Geometry check sheet. Reference: the model listing, model coordinates, mm. Face numbers are marked on the shaded views. A direction names the side the tool comes from. Give positions to 0.01 mm unless a question says otherwise; leave off trailing zeros. Write each loop counter-clockwise with the first axis right and the second up, starting at its lowest first coordinate (ties: lowest second). Pieces come first, ordered by that corner, then holes.
(1) Tool access check on the marked faces 1 and 2. Record the directions out of +Z, -Z, +X, -X, +Y, -Y that give a thin tool (end or side, any length) a straight path to the whole face; none if there is none.
(2) Thickness scan on line 1 along Y through (x, z) = (-10, -2); line 2 along X through (y, z) = (15, -73); line 3 along Z through (x, y) = (-15, 9.5). Record the ranges inside material, lowest first.
(3) Depth check by flat-ended pin: P1, Ø4, axis at x = -10, y = 10, coming from the -Z side; P2, Ø3, axis at y = 9.5, z = -33, coming from the +X side; P3, Ø12, axis at y = 9.5, z = -52.5, coming from the -X side; P4, Ø7, axis at x = -8, y = 11, coming from the -Z side. Enter the tip coordinate at first touch or a pass-through.
(4) Cross-section at B-B (x = -10). Record the boundary of the cut face in (y, z), and give its area (3 significant figures).
(5) Cross-section at D-D (x = 4). Record the boundary of the cut face in (y, z).
(6) Cross-section at C-C (z = -6). Record the boundary of the cut face in (x, y).
(7) Cross-section at A-A (y = 10). Record the boundary of the cut face in (x, z).
```python
from build123d import *

# Parameters (mm, degrees)
BOSS_EXTRUDE1_DEPTH = 20
SKETCH2_R           = 2.65
CUT_EXTRUDE1_DEPTH  = 20
SKETCH3_R           = 2.65
CUT_EXTRUDE2_DEPTH  = 20
SKETCH7_R           = 6
CUT_EXTRUDE4_DEPTH  = 5
SKETCH8_R           = 6
CUT_EXTRUDE5_DEPTH  = 5
CHAMFER3_SIZE       = 4
FILLET2_R           = 4
CHAMFER4_SIZE       = 2
CHAMFER5_SIZE       = 1


with BuildPart() as part:
    # Sketch1 → Boss-Extrude1 (new body)
    with BuildSketch(Plane(origin=(0, 0, 0), x_dir=(1, 0, 0), z_dir=(0, 1, 0))):
        with BuildLine():
            Line((-4.142135624, 0), (-20, 0))
            Line((-20, 0), (-20, 10))
            Line((-20, 10), (-8.284271247, 10))
            ThreePointArc((-8.284271247, 10), (-4.457436924, 10.761204675), (-1.213203436, 12.928932188))
            Line((-1.213203436, 12.928932188), (43.639610307, 57.781745931))
            ThreePointArc((43.639610307, 57.781745931), (45.80733782, 61.025979419), (46.568542495, 64.852813742))
            Line((46.568542495, 64.852813742), (46.568542495, 76.568542495))
            Line((46.568542495, 76.568542495), (56.568542495, 76.568542495))
            Line((56.568542495, 76.568542495), (56.568542495, 60.710678119))
            ThreePointArc((56.568542495, 60.710678119), (55.80733782, 56.883843795), (53.639610307, 53.639610307))
            Line((53.639610307, 53.639610307), (2.928932188, 2.928932188))
            ThreePointArc((2.928932188, 2.928932188), (-0.3153013, 0.761204675), (-4.142135624, 0))
        make_face()
    extrude(amount=BOSS_EXTRUDE1_DEPTH)

    # Sketch2 → Cut-Extrude1 (cut)
    with BuildSketch(Plane.XY):
        with Locations((-10, 10)):
            Circle(SKETCH2_R)
    extrude(amount=-CUT_EXTRUDE1_DEPTH, mode=Mode.SUBTRACT)

    # Sketch3 → Cut-Extrude2 (cut)
    with BuildSketch(Plane(origin=(56.568542495, 0, 0), x_dir=(0, 0, -1), z_dir=(1, 0, 0))):
        with Locations((66.568542495, 10)):
            Circle(SKETCH3_R)
    extrude(amount=-CUT_EXTRUDE2_DEPTH, mode=Mode.SUBTRACT)

    # Sketch7 → Cut-Extrude4 (cut)
    with BuildSketch(Plane.ZY.offset(-46.568542495)):
        with Locations((-66.568542495, 10)):
            Circle(SKETCH7_R)
    extrude(amount=CUT_EXTRUDE4_DEPTH, mode=Mode.SUBTRACT)

    # Sketch8 → Cut-Extrude5 (cut)
    with BuildSketch(Plane(origin=(0, 0, -10), x_dir=(-1, 0, 0), z_dir=(0, 0, -1))):
        with Locations((10, 10)):
            Circle(SKETCH8_R)
    extrude(amount=CUT_EXTRUDE5_DEPTH, mode=Mode.SUBTRACT)

    # Chamfer3
    chamfer3_edges = [part.edges().sort_by_distance(p)[0] for p in [
        (51.568542495, 0, -76.568542495),
        (-20, 0, -5),
        (51.568542495, 20, -76.568542495),
        (-20, 20, -5),
    ]]
    chamfer(chamfer3_edges, length=CHAMFER3_SIZE)

    # Fillet2
    fillet2_edges = [part.edges().sort_by_distance(p)[0] for p in [
        (-16, 20, -5),
        (51.568542495, 20, -72.568542495),
        (51.568542495, 4, -76.568542495),
        (51.568542495, 16, -76.568542495),
        (-16, 0, -5),
        (51.568542495, 0, -72.568542495),
        (-20, 16, -5),
        (-20, 4, -5),
    ]]
    fillet(fillet2_edges, radius=FILLET2_R)

    # Chamfer4
    chamfer4_edges = [part.edges().sort_by_distance(p)[0] for p in [
        (46.568542495, 20, -67.882250994),
        (46.568542495, 18, -74.568542495),
        (46.568542495, 2, -74.568542495),
        (46.568542495, 0, -67.882250994),
        (46.568542495, 15.87387948, -76.264060625),
        (46.568542495, 19.69551813, -72.442421975),
        (46.568542495, 0.30448187, -72.442421975),
        (46.568542495, 4.12612052, -76.264060625),
        (-18, 18, -10),
        (-11.313708499, 0, -10),
        (-18, 2, -10),
        (-20, 10, -10),
        (-19.69551813, 4.12612052, -10),
        (-15.87387948, 0.30448187, -10),
        (-19.69551813, 15.87387948, -10),
        (-15.87387948, 19.69551813, -10),
        (-4.457436924, 0, -10.761204675),
        (21.213203436, 0, -35.355339059),
        (45.80733782, 0, -61.025979419),
        (45.80733782, 20, -61.025979419),
        (21.213203436, 20, -35.355339059),
        (-4.457436924, 20, -10.761204675),
        (-11.313708499, 20, -10),
        (46.568542495, 10, -76.568542495),
    ]]
    chamfer(chamfer4_edges, length=CHAMFER4_SIZE)

    # Chamfer5
    chamfer5_edges = [part.edges().sort_by_distance(p)[0] for p in [
        (56.568542495, 2, -74.568542495),
        (56.568542495, 18, -74.568542495),
        (56.568542495, 15.87387948, -76.264060625),
        (56.568542495, 19.69551813, -72.442421975),
        (56.568542495, 0.30448187, -72.442421975),
        (56.568542495, 4.12612052, -76.264060625),
        (-9.242640687, 0, 0),
        (-9.242640687, 20, 0),
        (-20, 10, 0),
        (-18, 2, 0),
        (-18, 18, 0),
        (-19.69551813, 4.12612052, 0),
        (-15.87387948, 0.30448187, 0),
        (-19.69551813, 15.87387948, 0),
        (-15.87387948, 19.69551813, 0),
        (-0.3153013, 20, -0.761204675),
        (56.568542495, 0, -65.811183182),
        (55.80733782, 0, -56.883843795),
        (28.284271247, 0, -28.284271247),
        (-0.3153013, 0, -0.761204675),
        (28.284271247, 20, -28.284271247),
        (55.80733782, 20, -56.883843795),
        (56.568542495, 20, -65.811183182),
        (56.568542495, 10, -76.568542495),
    ]]
    chamfer(chamfer5_edges, length=CHAMFER5_SIZE)


solid = part.part
```
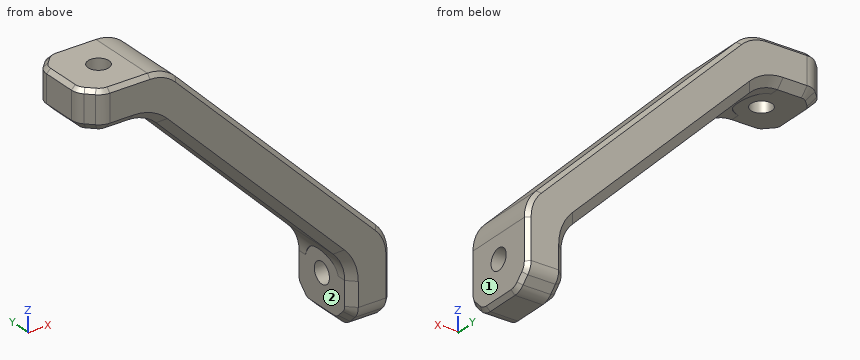
Reply:
1. face 1: +Z, -Z, +X, +Y, -Y
1. face 2: -Z, -X
2. line 1: y = 0 to 7.35, 12.65 to 20
2. line 2: x = 46.57 to 56.57
2. line 3: z = -10 to 0
3. P1: passes through
3. P2: stops at x = 34.5
3. P3: stops at x = 32.36
3. P4: stops at z = -10
4. outline: (0, -8) - (2, -10) - (7.35, -10) - (7.35, 0) - (1, 0) - (0, -1) - close; (12.65, -10) - (18, -10) - (20, -8) - (20, -1) - (19, 0) - (12.65, 0) - close
4. area: 142 mm2
5. outline: (0, -15.31) - (2, -18.14) - (18, -18.14) - (20, -15.31) - (20, -5.41) - (19, -4) - (1, -4) - (0, -5.41) - close
6. outline: (-20, 5.66) arc R4 ccw to (-18.83, 2.83) - (-17.17, 1.17) arc R4 ccw to (-14.34, 0) - (4.59, 0) - (6, 1) - (6, 19) - (4.59, 20) - (-14.34, 20) arc R4 ccw to (-17.17, 18.83) - (-18.83, 17.17) arc R4 ccw to (-20, 14.34) - close; hole circle Ø5.3 at (-10, 10)
7. outline: (-20, -8) - (-18, -10) - (-12.65, -10) - (-12.65, 0) - (-19, 0) - (-20, -1) - close; (-7.35, -10) - (-4, -10) - (-4, -10.96) arc R10 cw to (-1.21, -12.93) - (43.64, -57.78) arc R10 cw to (45.6, -60.57) - (46.57, -60.57) - (46.57, -63.92) - (56.57, -63.92) - (56.57, -60.71) arc R10 ccw to (53.64, -53.64) - (2.93, -2.93) arc R10 ccw to (-4.14, 0) - (-7.35, 0) - close; (46.57, -74.57) - (48.57, -76.57) - (55.57, -76.57) - (56.57, -75.57) - (56.57, -69.22) - (46.57, -69.22) - close
